Could you check a few things on this drawing? It's one solid part, dimensions in mm from its lowest x, y, z. Coordinates: 2 decimals unless noted, no trailing zeros. Order: outer loops, then holes, each group sorted by start corner. A loop starts at its lowest first (then second) coordinate and runs counter-clockwise, first axis right, second up. Notation, with made-up numbers: (29, 20) -> (73, 20) arc R27 ccw to (73, 43) -> close; hole circle Ø9 at (50, 21.5). An arc over 180 degrees is marked (long way). Use a Markdown table: item, result. Add a question column.
1. Suppose I cut it at B-B, the plane x = 2. List the corners of the cut face in (y, z) for me.
2. Suppose I cut it at A-A, the plane y = 73. List the corners of the cut face in (x, z) for me.
3. For pin 1 Ø1 at (y, z) = (23, 2) entering from +X, with a flat end and sliding along its axis, tell me the tip position at first contact or that it passes through.
4. If I drill on line 1 along X through (y, z) = (73, 1.1); line 2 along Y through (x, z) = (2, 1.25); line 3 along Z through (x, y) = (0.4, 71), over which ranges is the centre line in solid material (lowest first)? Write a range as from..to.
5. Suppose I cut it at C-C, the plane y = 16. List the corners of the cut face in (x, z) for me.
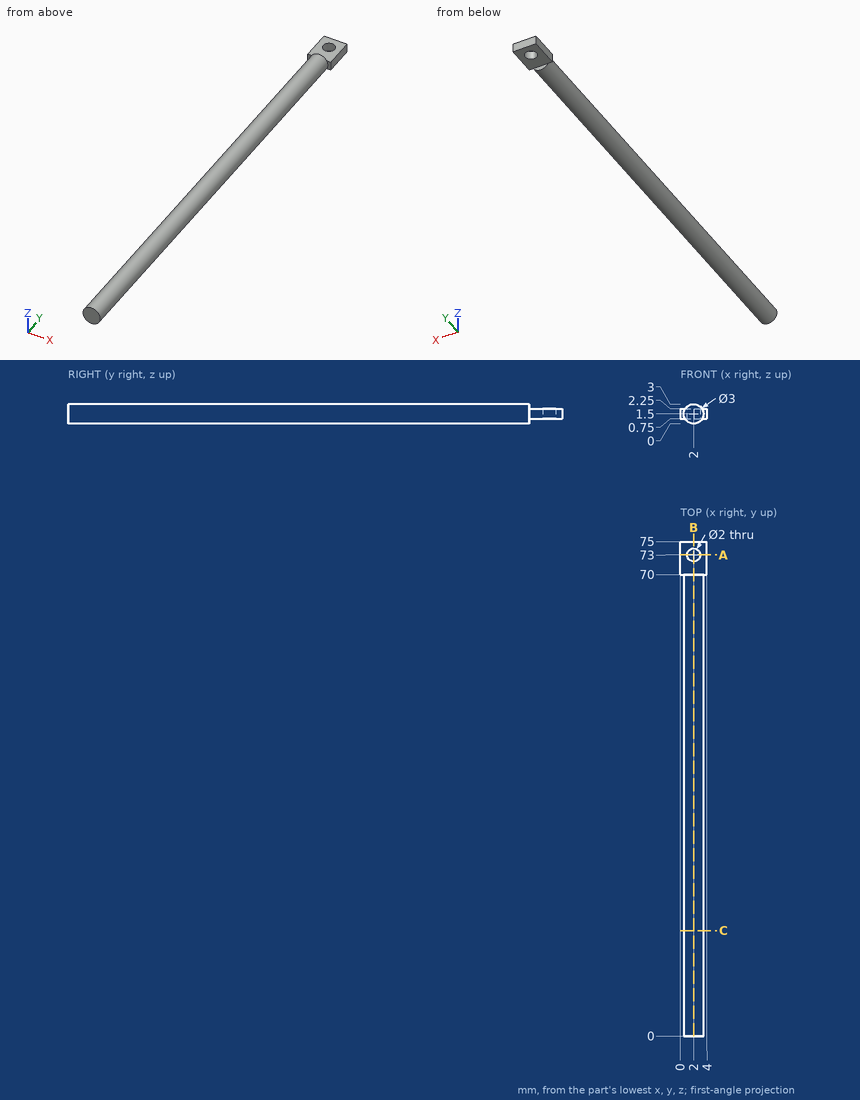
Worked out:
| question | item | result |
|---|---|---|
| 1 | outline | (0, 0) -> (70, 0) -> (70, 0.75) -> (72, 0.75) -> (72, 2.25) -> (70, 2.25) -> (70, 3) -> (0, 3) -> close; (74, 0.75) -> (75, 0.75) -> (75, 2.25) -> (74, 2.25) -> close |
| 2 | outline | (0, 0.75) -> (1, 0.75) -> (1, 2.25) -> (0, 2.25) -> close; (3, 0.75) -> (4, 0.75) -> (4, 2.25) -> (3, 2.25) -> close |
| 3 | pin 1 | stops at x = 3.5 |
| 4 | line 1 | x = 0..1, 3..4 |
| 4 | line 2 | y = 0..72, 74..75 |
| 4 | line 3 | z = 0.75..2.25 |
| 5 | outline | circle Ø3 at (2, 1.5) |
